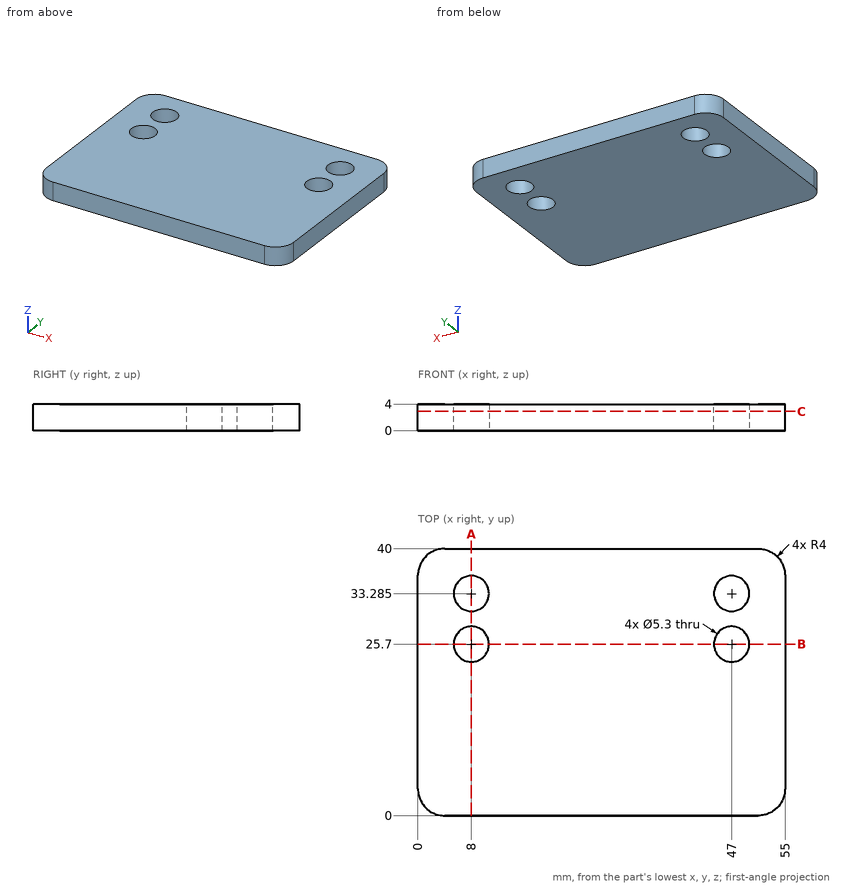
Design review of the part shown in the three views and the two pictorial views. Dimensions are in mm from the part's minimum x, y and z. Coordinates: 2 decimals unless noted, no trailing zeros. Loops run counter-clockwise (first coordinate to the right, second up) from the corner with the lowest first, then second, coordinate; pieces in that order, holes last. Notation, with made-up numbers: (-10, 26) -> (29, 26) arc R10 cw to (29, 39) -> close; hole circle Ø11 at (39.5, -12). An arc over 180 degrees is marked (long way). Answer as CSV lines item,"result".
Item 1: Take a section at C-C, the plane z = 2.9. State the section outline as (x, y) points (3 decimals), and give its area (3 significant figures).
Results below:
outline,"(0, 4) arc R4 ccw to (4, 0) -> (51, 0) arc R4 ccw to (55, 4) -> (55, 36) arc R4 ccw to (51, 40) -> (4, 40) arc R4 ccw to (0, 36) -> close; hole circle Ø5.3 at (8, 25.7); hole circle Ø5.3 at (8, 33.285); hole circle Ø5.3 at (47, 25.7); hole circle Ø5.3 at (47, 33.285)"
area,"2,100 mm2"
Item 2: Take a section at A-A, the plane x = 8. State the section outline as (y, z) points (3 decimals).
Results below:
outline,"(0, 0) -> (23.05, 0) -> (23.05, 4) -> (0, 4) -> close; (28.35, 0) -> (30.635, 0) -> (30.635, 4) -> (28.35, 4) -> close; (35.935, 0) -> (40, 0) -> (40, 4) -> (35.935, 4) -> close"
Item 3: For L1, parallel to Y at x = 8, z = 2.85 (3 decimals); L2, parallel to Y at x = 3, z = 2.4; L3, parallel to X at y = 2.5, z = 1.8, list the stretches that pass through material, from the lowest coordinate up.
Results below:
L1,"y = 0 to 23.05, 28.35 to 30.635, 35.935 to 40"
L2,"y = 0.13 to 39.87"
L3,"x = 0.29 to 54.71"
Item 4: Take a section at B-B, the plane y = 25.7. State the section outline as (x, z) points, and give its area (3 significant figures).
Results below:
outline,"(0, 0) -> (5.35, 0) -> (5.35, 4) -> (0, 4) -> close; (10.65, 0) -> (44.35, 0) -> (44.35, 4) -> (10.65, 4) -> close; (49.65, 0) -> (55, 0) -> (55, 4) -> (49.65, 4) -> close"
area,"178 mm2"
